```python
from build123d import *

# Parameters (mm, degrees)
F1_DEPTH = 25
F2_W     = 40
F2_H     = 12.5
F3_DEPTH = 35
F5_DEPTH = 25
F6_DEPTH = 5


with BuildPart() as f1:
    # F0 (on Top) → F1 (new body)
    with BuildSketch(Plane.XY):
        with BuildLine():
            ThreePointArc((17.5, -6), (0, -18.5), (-17.5, -6))
            Line((-17.5, -6), (-20, -6))
            Line((-20, -6), (-20, -31))
            Line((-20, -31), (20, -31))
            Line((20, -31), (20, -6))
            Line((20, -6), (17.5, -6))
        make_face()
    extrude(amount=F1_DEPTH)

    # F2 (on face) → F3 (join)
    with BuildSketch(Plane(origin=(0, 0, 0), x_dir=(1, 0, 0), z_dir=(0, 0, -1))):
        with Locations((0, 24.75)):
            Rectangle(F2_W, F2_H)
    extrude(amount=F3_DEPTH)

    # F4 (on face) → F5 (join)
    with BuildSketch(Plane(origin=(0, 0, -35), x_dir=(1, 0, 0), z_dir=(0, 0, -1))):
        with BuildLine():
            Line((-20, 6), (-17.5, 6))
            ThreePointArc((-17.5, 6), (-10.7529065838, 15.0540692173), (0, 18.5))
            Line((0, 18.5), (-20, 18.5))
            Line((-20, 18.5), (-20, 6))
        make_face()
        Polygon((-20, 18.5), (0, 18.5), (20, 18.5), (20, 31), (-20, 31), align=None)
        with BuildLine():
            ThreePointArc((0, 18.5), (10.7529065838, 15.0540692173), (17.5, 6))
            Line((17.5, 6), (20, 6))
            Line((20, 6), (20, 18.5))
            Line((20, 18.5), (0, 18.5))
        make_face()
    extrude(amount=F5_DEPTH)

    # F6 (cut): a face of the model
    f6_faces = [f1.faces().sort_by_distance(p)[0] for p in [
        (0, -18.5, -17.5),
    ]]
    extrude(f6_faces, amount=-F6_DEPTH, mode=Mode.SUBTRACT)


solid = f1.part
```
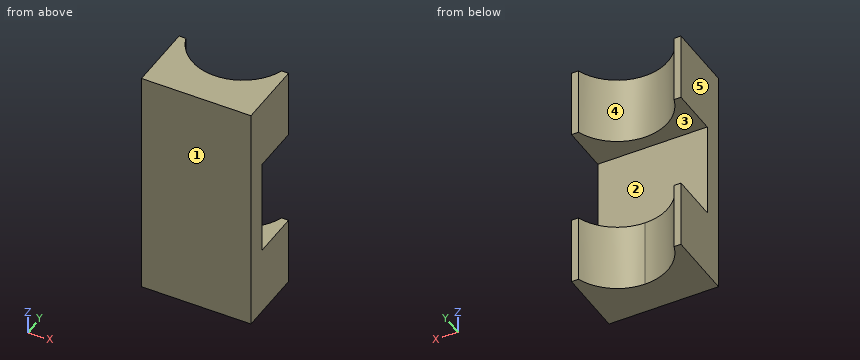
The model under review builds one solid part; all positions refer to its coordinate system, in mm. Face numbers are marked on the shaded views. A direction names the side the tool comes from. Round coordinates to 2 decimals unless told otherwise and drop trailing zeros. Write each loop counter-clockwise with the first axis right and the second up, starting at its lowest first coordinate (ties: lowest second). Pieces come first, ordered by that corner, then holes. Notation, with made-up numbers: (33.25, -39.5) -> (41.25, -39.5) arc R32 cw to (41.25, -5.5) -> close; hole circle Ø9 at (44, 49.5). An arc over 180 degrees is marked (long way). Use CSV: the item, a comma, the result in double quotes.
Q1. To check wall thickness, follow probe 1 along Z at (x, y) = (-9.5, -17.25); probe 2 along Y at (x, z) = (-15, -9); probe 3 along X at (y, z) = (-10, 18.5). State the ranges of each line that lie inside material, in increasing order. Write a range as [from, to].
Checks:
probe 1,"[-60, -35], [0, 25]"
probe 2,"[-31, -23.5]"
probe 3,"[-20, -15.56], [15.56, 20]"
Q2. For pin 1 Ø10.5 at (x, z) = (3, -26) entering from +Y; pin 2 Ø4 at (y, z) = (-20, -4.5) entering from -X, all flat-tipped, find the tip position at first contact; note any pin that passes through.
Checks:
pin 1,"y = -23.5"
pin 2,"through"
Q3. Consider section B-B (x = 14.5). Give the boundary of the cut face in (y, z), then the cut area to 3 significant figures.
Checks:
outline,"(-31, -60) -> (-11.49, -60) -> (-11.49, -35) -> (-23.5, -35) -> (-23.5, 0) -> (-11.49, 0) -> (-11.49, 25) -> (-31, 25) -> close"
area,"1,240 mm²"
Q4. Consider section C-C (z = 5.5). Give the boundary of the cut face in (x, y), then the cut area to 3 significant figures.
Checks:
outline,"(-20, -31) -> (20, -31) -> (20, -6) -> (17.5, -6) arc R18.5 cw to (-17.5, -6) -> (-20, -6) -> close"
area,"680 mm²"
Q5. Consider section A-A (y = -21.5). Give the boundary of the cut face in (x, z).
Checks:
outline,"(-20, -60) -> (20, -60) -> (20, -35) -> (-20, -35) -> close; (-20, 0) -> (20, 0) -> (20, 25) -> (-20, 25) -> close"
Q6. For the marked faces 1 and 2, list the 3-axis set-ups (+Z, -Z, +X, -X, +Y, -Y) from which the entire face can be reached by the end or side of a thin tool; tool diameter is ignored.
Checks:
face 1,"+Z, -Z, +X, -X, -Y"
face 2,"+X, -X, +Y"
Q7. Mouldability with a two-part tool opening along X and no side actions: class the marked faces 3, 4 and 5 as released by +X, released by -X, zero draft, split by the parting line, or undercut.
Checks:
face 3,"zero draft"
face 4,"undercut"
face 5,"released by -X"
Q8. Consider section D-D (x = -15). Give the boundary of the cut face in (y, z), then the cut area to 3 significant figures.
Checks:
outline,"(-31, -60) -> (-10.83, -60) -> (-10.83, -35) -> (-23.5, -35) -> (-23.5, 0) -> (-10.83, 0) -> (-10.83, 25) -> (-31, 25) -> close"
area,"1,270 mm²"
